Autodesk Inventor part; units mm, degrees
ref_plane "YZ Plane" through (0, 0, 0) normal (1, 0, 0) x (0, 1, 0)
ref_plane "XZ Plane" through (0, 0, 0) normal (0, 1, 0) x (-1, 0, 0)
ref_plane "XY Plane" through (0, 0, 0) normal (0, 0, 1) x (1, 0, 0)
sketch "Sketch1" plane through (0, 0, 0) normal (0, 1, 0) x (-1, 0, 0)
  circle A0 centre (0, 0) radius 26.1938
  circle A1 centre (0, 0) radius 19.05
  dimension "d0" = 52.3875
  dimension "d1" = 38.1
extrude "Extrusion1" add sketch "Sketch1" along normal blind 3.175
sketch "Sketch2" plane through (0, 0, 0) normal (0, 0, 1) x (1, 0, 0)
  line L0 (-21.8281, 0) -> (-21.8281, -1.5875)
  circle A0 centre (-21.8281, -1.5875) radius 2.7781
  line L1 (0, 0) -> (0, 3.175)
  line L2 (26.1938, 3.175) -> (-26.1938, 3.175)
  dimension "d4" = 1.5875
  dimension "d5" = 5.5563
revolve "Revolution1" cut sketch "Sketch2" angle 360 about axis through (0, 0, 0) along (0, 1, 0)
chamfer "Chamfer1" distance 0.3969 angle 45 1 edges at (26.1938, 3.175, 0)
chamfer "Chamfer2" distance 0.3969 angle 45 1 edges at (26.1938, 0, 0)
chamfer "Chamfer3" distance 0.3969 angle 45 1 edges at (19.05, 3.175, 0)
properties part number "ThrustBearing-UpperRing"
Input: part model. Units: mm. Frame: model coordinates. Round coordinates to 2 decimals unless told otherwise and drop trailing zeros. Loops run counter-clockwise (first coordinate to the right, second up) from the corner with the lowest first, then second, coordinate; pieces in that order, holes last.
1) Pin query (flat end, axial travel): pin 1 (1 mm diameter, centred on x = -15, y = 2.5, fed in from -Z); pin 2 (23 mm diameter, centred on x = 0, z = 0, fed in from +Y). Return the tip coordinate at first contact, or that it passes through.
Ans:
pin 1: stops at z = -21.81
pin 2: passes through
2) Material intervals for line 1 (Z direction, x = 0, y = 0.75); line 2 (X direction, y = 0.75, z = -11); line 3 (Z direction, x = 0, y = 1.55), sorted ascending.
Ans:
line 1: z = -26.19 to -23.33, -20.33 to -19.05, 19.05 to 20.33, 23.33 to 26.19
line 2: x = -23.77 to -20.57, -17.09 to -15.55, 15.55 to 17.09, 20.57 to 23.77
line 3: z = -26.19 to -19.05, 19.05 to 26.19
3) Section query C-C on y = 1.85. Return the cut outline in (x, z), plus the area to 3 significant figures.
Ans:
outline: circle Ø52.39 at (0, 0); hole circle Ø38.1 at (0, 0)
area: 1,020 mm2
4) Pull-direction query (Z, two-part tool) for faces 1 (the cylindrical face through (3.41, 1.57, -25.97)), 2 (the cylindrical face through (15.12, 1.37, 11.59)), 3 (the flat face through (10, 3.175, 17)); classes: released by +Z, released by -Z, zero draft, split by the parting line, or undercut.
Ans:
face 1: split by the parting line
face 2: undercut
face 3: zero draft
